Geometry check sheet. Reference: drawing and pictorial views, mm from the part's lowest x, y, z. Give positions to 0.01 mm unless a question says otherwise; leave off trailing zeros. Loops run counter-clockwise (first coordinate to the right, second up) from the corner with the lowest first, then second, coordinate; pieces in that order, holes last. Notation, with made-up numbers: (79.5, 77.25) - (100.5, 77.25) arc R26 cw to (100.5, 111.25) - close; hole circle Ø3 at (6.5, -0.75). An arc over 180 degrees is marked (long way). Use CSV: the item, a comma, the result in double quotes.
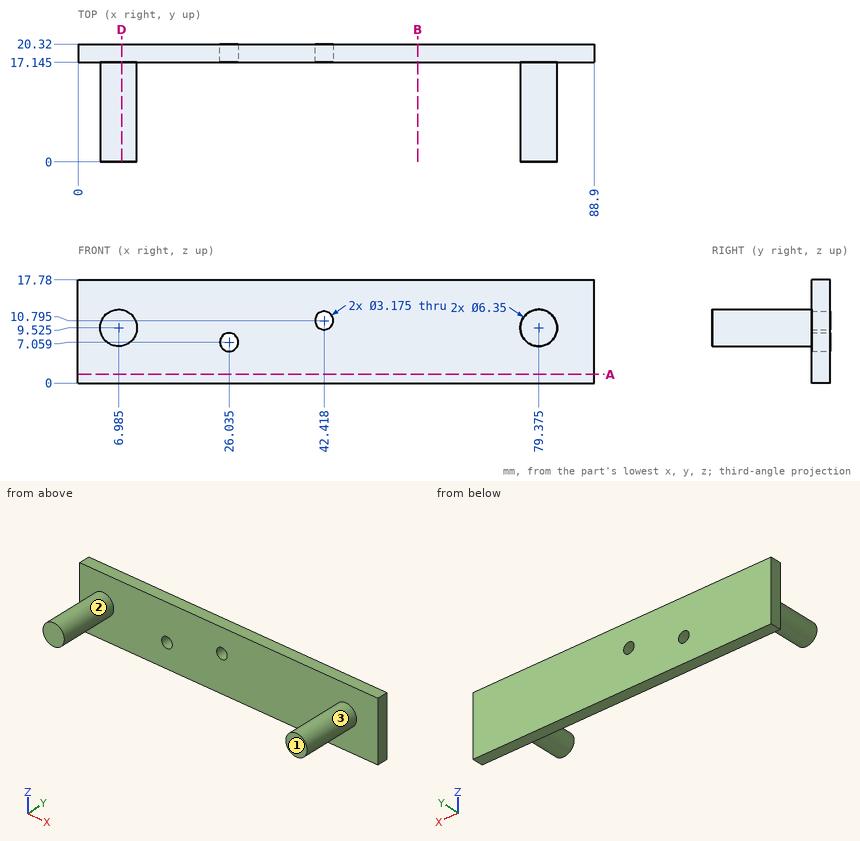
1. Go/stop test with flat-tipped pins: pin 1 Ø1 at (x, z) = (31.5, 2.5) entering from -Y (3 decimals); pin 2 Ø8 at (y, z) = (11, 6) entering from -X; pin 3 Ø4 at (y, z) = (13.5, 15) entering from +X. Record where each tip stops, or that it passes through.
Completed:
pin 1,"stops at y = 17.145"
pin 2,"stops at x = 3.81"
pin 3,"passes through"
2. Sectioned sample at A-A, the plane z = 1.5. Record the boundary of the cut face in (x, y) (1 decimal).
Completed:
outline,"(0, 17.1) - (88.9, 17.1) - (88.9, 20.3) - (0, 20.3) - close"
3. Scan lines: line 1 along X through (y, z) = (7, 9.25); line 2 along Y through (x, z) = (32, 13.25) (1 decimal); line 3 along X through (y, z) = (2.75, 11.5). Record each from-to range of solid material in increasing order.
Completed:
line 1,"x = 3.82 to 10.15, 76.21 to 82.54"
line 2,"y = 17.1 to 20.3"
line 3,"x = 4.5 to 9.47, 76.89 to 81.86"
4. Sectioned sample at B-B, the plane x = 58.5. Record the boundary of the cut face in (y, z) (1 decimal).
Completed:
outline,"(17.1, 0) - (20.3, 0) - (20.3, 17.8) - (17.1, 17.8) - close"
5. Sectioned sample at D-D, the plane x = 7.5. Record the boundary of the cut face in (y, z) (1 decimal), and give its area (3 significant figures).
Completed:
outline,"(0, 6.4) - (17.1, 6.4) - (17.1, 0) - (20.3, 0) - (20.3, 17.8) - (17.1, 17.8) - (17.1, 12.7) - (0, 12.7) - close"
area,"164 mm²"
6. Release check for a two-part mould opening along X. For the marked faces 1, 2 and 3 record: released by +X, released by -X, zero draft, split by the parting line, or undercut.
Completed:
face 1,"zero draft"
face 2,"undercut"
face 3,"undercut"
